CAD build for the part. Positions are in the model's coordinates, mm. Give positions to 0.01 mm unless a question says otherwise; leave off trailing zeros. Write each loop counter-clockwise with the first axis right and the second up, starting at its lowest first coordinate (ties: lowest second). Pieces come first, ordered by that corner, then holes. Notation, with made-up numbers: M -33,36 L -4,36 A18 cw -4,43 Z; hole C -20.5,15.5 d8. An arc over 180 degrees is marked long. One line per question, with ' | ' between items. Start each with the question number.
1. Cut at A-A, the plane y = 0. Write the cut outline in (x, z).
2. Wall check: L1, parallel to Y at x = 0, z = 6; L2, parallel to Z at x = 3.5, y = 3.25; L3, parallel to X at y = -8.5, z = 9.75. Give the ranges that are in metal, low to high.
3. Pull direction X, two halves, no side cores. Call faces 1 (the face through (11, -4, 0)), 2 (the face through (-1.5, 11.4, 7.6)), 3 (the face through (11.923, 3.755, 7.642)), 4 (the face through (5, 0, 16.5)): released by +X, released by -X, zero draft, split by the parting line, or undercut.
4. Flat gauge pins, fed straight in: pin 1 (3 mm diameter, centred on y = 10, z = 5, fed in from +X); pin 2 (1.5 mm diameter, centred on x = -8.5, z = 14.5, fed in from -Y); pin 3 (2 mm diameter, centred on x = 3.5, z = 10, fed in from +Y). Where does each tip first touch, or does it go through?
5. Cut at C-C, the plane z = 13. Write the cut outline in (x, y), then the cut area to 3 significant figures.
```python
from build123d import *

# Parameters (mm, degrees)
SKETCH8_R      = 12.5
EXTRUDE6_DEPTH = 17.5
FILLET2_R      = 2
SHELL1_T       = -1
SKETCH9_R      = 4
EXTRUDE7_DEPTH = 25.874685978


with BuildPart() as part:
    # Sketch8 → Extrude6 (new body)
    with BuildSketch(Plane.XY):
        Circle(SKETCH8_R)
    extrude(amount=EXTRUDE6_DEPTH)

    # Fillet2
    fillet2_edges = [part.edges().sort_by_distance(p)[0] for p in [
        (-12.5, 0, 17.5),
    ]]
    fillet(fillet2_edges, radius=FILLET2_R)

    # Shell1
    shell1_openings = [part.faces().sort_by_distance(p)[0] for p in [
        (0, 0, 0),
    ]]
    offset(amount=SHELL1_T, openings=shell1_openings, kind=Kind.INTERSECTION)

    # Sketch9 → Extrude7 (cut, through all)
    with BuildSketch(Plane.XY.offset(17.5)):
        Circle(SKETCH9_R)
    extrude(amount=-EXTRUDE7_DEPTH, mode=Mode.SUBTRACT)


solid = part.part
```
Here are the results:
1) outline: M -12.5,0 L -11.5,0 L -11.5,15.5 A1 cw -10.5,16.5 L -4,16.5 L -4,17.5 L -10.5,17.5 A2 ccw -12.5,15.5 Z; M 4,16.5 L 10.5,16.5 A1 cw 11.5,15.5 L 11.5,0 L 12.5,0 L 12.5,15.5 A2 ccw 10.5,17.5 L 4,17.5 Z
2) L1: -12.5 to -11.5, 11.5 to 12.5 | L2: 16.5 to 17.5 | L3: -9.17 to -7.75, 7.75 to 9.17
3) face 1: zero draft | face 2: undercut | face 3: split by the parting line | face 4: undercut
4) pin 1: x = 9.17 | pin 2: y = -9.81 | pin 3: y = 12.25
5) outline: C 0,0 d25; hole C 0,0 d23 | area: 75.4 mm^2
